from build123d import *

# Parameters (mm, degrees)
SKETCH1_R           = 2.5
BOSS_EXTRUDE1_DEPTH = 5


with BuildPart() as part:
    # Sketch1 → Boss-Extrude1 (new body)
    with BuildSketch(Plane(origin=(0, 0, 0), x_dir=(1, 0, 0), z_dir=(0, 1, 0))):
        with BuildLine():
            ThreePointArc((-1.35433299, -25.15), (0.768377165, -28.682107422), (4.88355843, -28.465394696))
            Line((4.88355843, -28.465394696), (22.88355843, -16.315394696))
            ThreePointArc((22.88355843, -16.315394696), (24.645161473, -12.936407261), (22.777022974, -9.615133422))
            Line((22.777022974, -9.615133422), (2.131355964, 3.384866578))
            ThreePointArc((2.131355964, 3.384866578), (-1.933206681, 3.501815519), (-4, 0))
            Line((-4, 0), (-1.35433299, -25.15))
        make_face()
        with Locations(Location((2.64566701, -25.15, 0), (0, 0, 270))):
            Circle(SKETCH1_R, mode=Mode.SUBTRACT)
        with Locations(Location((20.64566701, -13, 0), (0, 0, 270))):
            Circle(SKETCH1_R, mode=Mode.SUBTRACT)
        with Locations(Location((0, 0, 0), (0, 0, 270))):
            Circle(SKETCH1_R, mode=Mode.SUBTRACT)
    extrude(amount=BOSS_EXTRUDE1_DEPTH)


solid = part.part
Can you work these out from the model? Positions are in its coordinate system, mm. Give positions to 0.01 mm unless a question says otherwise; leave off trailing zeros. Loops run counter-clockwise (first coordinate to the right, second up) from the corner with the lowest first, then second, coordinate; pieces in that order, holes last. Notation, with made-up numbers: M 2,17 L 56,17 A24 cw 56,47 Z; hole C 11,-29 d9. An arc over 180 degrees is marked long. One line per item, written item: value. Start each with the question number.
1) If we section it at C-C, the plane z = -1: Write out the boundary of the cut face in (x, y).
2) Thinking about a two-plate mould opening in X: for faces 1 (the face through (7, 0, 12)), 2 (the face through (0.715, 2.465, 28.653)), 3 (the face through (19.12, 2.46, 11.02)), which applies, +X half, -X half, draft (parallel to the pull), parting line (faces both ways), or undercut?
3) If we section it at D-D, the plane x = 13: Write out the boundary of the cut face in (y, z), and give its area (3 significant figures).
4) I'm going to push flat-ended pins straight in: pin 1 (1.5 mm diameter, centred on y = 2, z = 15.5, fed in from +X); pin 2 (3 mm diameter, centred on x = 10.5, y = 4, fed in from -Z). Where does each tip first touch, or does it pass through?
5) If I drill on line 1 (X direction, y = 4.05, z = 1.5); line 2 (X direction, y = 1.8, z = 0); line 3 (Z direction, x = 0.75, y = 3.1), over which ranges is the centre line in solid material (lowest first)? Write a range as [from, to].
6) If we section it at B-B, the plane y = 3.45: Write out the boundary of the cut face in (x, z), and give its area (3 significant figures).
7) If we section it at A-A, the plane z = 13: Write out the boundary of the cut face in (x, y).
Completed:
1. outline: M -3.87,0 L -2.29,0 L -2.29,5 L -3.87,5 Z; M 2.29,0 L 5.92,0 L 5.92,5 L 2.29,5 Z
2. face 1: draft
2. face 2: parting line
2. face 3: undercut
3. outline: M 0,3.46 L 5,3.46 L 5,22.99 L 0,22.99 Z
3. area: 97.6 mm^2
4. pin 1: stops at x = 24.24
4. pin 2: stops at z = 0.94
5. line 1: x = [-3.84, -2], [2, 9.89]
5. line 2: x = [-4, -2.5], [2.5, 7.51]
5. line 3: z = [-3.93, -2.38], [2.38, 23.52], [26.78, 28.67]
6. outline: M -4,0 A4 ccw 2.13,-3.38 L 22.78,9.62 A4 ccw 22.88,16.32 L 4.88,28.47 A4 ccw -1.35,25.15 Z; hole C 0,0 d5; hole C 2.65,25.15 d5; hole C 20.65,13 d5
6. area: 519 mm^2
7. outline: M -2.63,0 L 18.15,0 L 18.15,5 L -2.63,5 Z; M 23.15,0 L 24.65,0 L 24.65,5 L 23.15,5 Z
